Can you work these out from the model? Positions are in its coordinate system, mm. A direction names the side the tool comes from. Coordinates: 2 decimals unless noted, no trailing zeros. Loops run counter-clockwise (first coordinate to the right, second up) from the corner with the lowest first, then second, coordinate; pieces in that order, holes last.
```python
from build123d import *

# Parameters (mm, degrees)
F1_DEPTH  = 25.4
F2_R      = 12.7
F3_DEPTH  = 25.4
F4_R      = 12.7
F5_DEPTH  = 25.4
F6_W      = 25.4
F6_H      = 50.8
F7_DEPTH  = 76.2
F9_DEPTH  = 25.4
F11_DEPTH = 25.4
F13_DEPTH = 25.4


with BuildPart() as f1:
    # F0 (on Top) → F1 (new body)
    with BuildSketch(Plane.XY):
        with BuildLine():
            ThreePointArc((51.4803717834, -15.7496363992), (76.8803717834, 9.6503636008), (51.4803717834, 35.0503636008))
            Line((51.4803717834, 35.0503636008), (-50.1196282166, 35.0503636008))
            Line((-50.1196282166, 35.0503636008), (-50.1196282166, -15.7496363992))
            Line((-50.1196282166, -15.7496363992), (51.4803717834, -15.7496363992))
        make_face()
    extrude(amount=F1_DEPTH)

    # F2 (on face) → F3 (cut)
    with BuildSketch(Plane.XY.offset(25.4)):
        with Locations((0.6803717834, 9.6503636008)):
            Circle(F2_R)
    extrude(amount=-F3_DEPTH, mode=Mode.SUBTRACT)

    # F4 (on face) → F5 (cut)
    with BuildSketch(Plane.XY.offset(25.4)):
        with Locations((38.7803717834, 9.6503636008)):
            Circle(F4_R)
    extrude(amount=-F5_DEPTH, mode=Mode.SUBTRACT)

    # F6 (on face) → F7 (join)
    with BuildSketch(Plane.XY.offset(25.4)):
        with Locations((-37.4196282166, 9.6503636008)):
            Rectangle(F6_W, F6_H)
    extrude(amount=F7_DEPTH)

    # F8 (on face) → F9 (cut)
    with BuildSketch(Plane.YZ.offset(-24.7196282166)):
        with BuildLine():
            ThreePointArc((9.6503637335, 101.6), (27.6108758899, 94.1605121953), (35.0503636008, 76.2))
            Line((35.0503636008, 76.2), (35.0503636008, 101.6))
            Line((35.0503636008, 101.6), (9.6503637335, 101.6))
        make_face()
    extrude(amount=-F9_DEPTH, mode=Mode.SUBTRACT)

    # F10 (on face) → F11 (cut)
    with BuildSketch(Plane.YZ.offset(-24.7196282166)):
        with BuildLine():
            ThreePointArc((-15.7496363992, 76.2), (-8.31014861, 94.1605122734), (9.6503636892, 101.6))
            Line((9.6503636008, 101.6), (-15.7496363992, 101.6))
            Line((-15.7496363992, 101.6), (-15.7496363992, 76.2))
        make_face()
    extrude(amount=-F11_DEPTH, mode=Mode.SUBTRACT)

    # F12 (on face) → F13 (cut)
    with BuildSketch(Plane.YZ.offset(-24.7196282166)):
        with BuildLine():
            ThreePointArc((9.6503636892, 101.6), (3.0763598979, 100.7345159992), (-3.0496363992, 98.1970452561))
            Line((-3.0496363992, 98.1970452561), (-3.0496363992, 79.6029547439))
            Line((-3.0496363992, 79.6029547439), (-3.0496363992, 72.7970452561))
            ThreePointArc((-3.0496363992, 72.7970452561), (9.6503636008, 63.0519925088), (22.3503636008, 72.7970452561))
            Line((22.3503636008, 72.7970452561), (22.3503636008, 79.6029547439))
            Line((22.3503636008, 79.6029547439), (22.3503636008, 98.1970452561))
            ThreePointArc((22.3503636008, 98.1970452561), (16.2243674105, 100.7345159706), (9.6503637335, 101.6))
        make_face()
    extrude(amount=-F13_DEPTH, mode=Mode.SUBTRACT)


solid = f1.part
```
(1) Which directions (+Z, -Z, +X, -X, +Y, -Y) give clear straight access to the entire face, cutting with the end or side of a thin tool? Please do faces 1 (the flat face through (-37, 22.35, 85)), 2 (the cylindrical face through (-37.24, -12.44, 88.74)), 3 (the flat face through (-24.72, 9, 53)).
Check values:
face 1: +Z, +X, -X
face 2: +Z, +X, -X, -Y
face 3: +Z, +X, +Y, -Y
(2) I want a section at B-B on z = 69.5. Write out the boundary of the cut face in (x, y), then the cut area to 3 significant figures.
Check values:
outline: (-50.12, -15.75) - (-24.72, -15.75) - (-24.72, -1.66) - (-50.12, -1.66) - close; (-50.12, 20.96) - (-24.72, 20.96) - (-24.72, 35.05) - (-50.12, 35.05) - close
area: 716 mm2
(3) I want a section at A-A on x = -4. Write out the boundary of the cut face in (y, z).
Check values:
outline: (-15.75, 0) - (-2.16, 0) - (-2.16, 25.4) - (-15.75, 25.4) - close; (21.46, 0) - (35.05, 0) - (35.05, 25.4) - (21.46, 25.4) - close
(4) If I drill on probe 1 along X at (y, z) = (3, 28); probe 2 along Z at (x, y) = (54, -10); probe 3 along Y at (x, z) = (30, 22), over which ranges is the centre line in solid material (lowest first)?
Check values:
probe 1: x = -50.12 to -24.72
probe 2: z = 0 to 25.4
probe 3: y = -15.75 to 0.47, 18.83 to 35.05
(5) If we mould it in two halves opening along Y, with no side actions, what happens to faces 4 (the flat face through (-50.12, 9, 38)), 5 (the cylindrical face through (50.894, 13.465, 12.878)), 6 (the cylindrical face through (76.874, 9.092, 12.522))? For each: released by +Y, released by -Y, zero draft, split by the parting line, or undercut.
Check values:
face 4: zero draft
face 5: undercut
face 6: split by the parting line
(6) I'm going to push flat-ended pins straight in: pin 1 (3 mm diameter, centred on y = -1, z = 15.5, fed in from +X); pin 2 (1 mm diameter, centred on x = -12.5, y = 3.5, fed in from +Z); pin 3 (5 mm diameter, centred on y = 13.5, z = 65, fed in from +X). Where does each tip first touch, or does it pass through?
Check values:
pin 1: stops at x = 75.17
pin 2: stops at z = 25.4
pin 3: stops at x = -24.72
(7) I want a section at C-C on x = -33. Write out the boundary of the cut face in (y, z).
Check values:
outline: (-15.75, 0) - (35.05, 0) - (35.05, 76.2) arc R25.4 ccw to (22.35, 98.2) - (22.35, 72.8) arc R13.15 cw to (-3.05, 72.8) - (-3.05, 98.2) arc R25.4 ccw to (-15.75, 76.2) - close
(8) I want a section at D-D on y = 13. Write out the boundary of the cut face in (x, z), then the cut area to 3 significant figures.
Check values:
outline: (-50.12, 0) - (-11.57, 0) - (-11.57, 25.4) - (-24.72, 25.4) - (-24.72, 63.49) - (-50.12, 63.49) - close; (12.93, 0) - (26.53, 0) - (26.53, 25.4) - (12.93, 25.4) - close; (51.03, 0) - (76.66, 0) - (76.66, 25.4) - (51.03, 25.4) - close
area: 2,940 mm2
